Input: part model. Units: mm. Frame: model coordinates. A direction names the side the tool comes from. Coordinates: 2 decimals unless noted, no trailing zeros. Order: outer loops, then holes, each group sorted by start corner. A loop starts at its lowest first (then second) coordinate and runs counter-clockwise, first axis right, second up. Notation, with made-up numbers: (80.5, 32) - (139.5, 32) arc R36 ccw to (139.5, 67) - close; hole circle Ø10 at (61.25, 10). An arc over 180 degrees is marked (long way). Answer as CSV lines item,"result". Start each with the question number.
Item 1: Draft query along X for faces 6 (the cylindrical face through (-16.786, -0.592, 23.806)), 7 (the flat face through (-15, -1, 6.658)), 8 (the flat face through (-14.317, -1, 10)). Return one class per face: +X half, -X half, draft (parallel to the pull), parting line (faces both ways), or undercut.
Item 2: Section A-A (z = 11). Output: boundary loops of the cut face in (x, y).
Item 3: First-contact query: pin 1 (2 mm diameter, centred on y = -10.5, z = 27.5, fed in from +X); pin 2 (1 mm diameter, centred on x = -16.5, y = -1, fed in from +Z); pin 3 (1 mm diameter, centred on y = -0.5, z = 15, fed in from +X). Flat tips, straight axial feed; report the tip coordinate or a pass-through.
Item 4: Access query for faces 1 (the flat face through (-25, -1, 12.433)), 2 (the flat face through (-19, 0, 20)), 3 (the flat face through (-22.559, -1, 16)), 4 (the flat face through (-25, -1, 13.533)), 5 (the flat face through (-15.417, -1, 10)). Directions: +Z, -Z, +X, -X, +Y, -Y. A direction counts if a zero-diameter tool reaches every point of the face in a straight line with its end or side. Return the directions, or none.
Item 5: Section C-C (x = -23.25). Output: boundary loops of the cut face in (y, z).
Item 6: Material intervals for line 1 along X through (y, z) = (-1, 22.75); line 2 along X through (y, z) = (-1, 28.25); line 3 along Y through (x, z) = (-20.5, 22.5), sorted ascending.
Item 7: Section D-D (z = 22). Output: boundary loops of the cut face in (x, y).
Item 8: Section B-B (x = -18). Output: boundary loops of the cut face in (y, z), and give its area (3 significant figures).
from build123d import *

# Parameters (mm, degrees)
F1_DEPTH = 1.2
F2_R     = 0.267864
F3_DEPTH = 12.7


with BuildPart() as f1:
    # F0 (on Front) → F1 (new body)
    with BuildSketch(Plane.XZ):
        with BuildLine():
            Line((-22.558661, 13.532754), (-22.558661, 17.550706))
            ThreePointArc((-22.558661, 17.550706), (-20.646676, 18.025718), (-18.973681, 19.066109))
            ThreePointArc((-18.973681, 19.066109), (-17.31198, 18.043084), (-15.41748, 17.575431))
            Line((-15.41748, 17.575431), (-15.41748, 13.55748))
            Line((-15.41748, 13.55748), (-18.455535, 13.55748))
            Line((-18.455535, 13.55748), (-18.455535, 12.45748))
            Line((-18.455535, 12.45748), (-15.41748, 12.45748))
            Line((-15.41748, 12.45748), (-15.41748, 6.657985))
            Line((-15.41748, 6.657985), (-14.31748, 6.657985))
            Line((-14.31748, 6.657985), (-14.31748, 12.45748))
            Line((-14.31748, 12.45748), (-11.279425, 12.45748))
            Line((-11.279425, 12.45748), (-11.279425, 13.55748))
            Line((-11.279425, 13.55748), (-14.31748, 13.55748))
            Line((-14.31748, 13.55748), (-14.31748, 17.575431))
            ThreePointArc((-14.31748, 17.575431), (-9.043176, 26.336733), (-19.002461, 28.658661))
            ThreePointArc((-19.002461, 28.658661), (-28.940326, 26.294523), (-23.658661, 17.550706))
            Line((-23.658661, 17.550706), (-23.658661, 13.532754))
            Line((-23.658661, 13.532754), (-26.696716, 13.532754))
            Line((-26.696716, 13.532754), (-26.696716, 12.432754))
            Line((-26.696716, 12.432754), (-23.658661, 12.432754))
            Line((-23.658661, 12.432754), (-23.658661, 6.63326))
            Line((-23.658661, 6.63326), (-22.558661, 6.63326))
            Line((-22.558661, 6.63326), (-22.558661, 12.432754))
            Line((-22.558661, 12.432754), (-19.520607, 12.432754))
            Line((-19.520607, 12.432754), (-19.520607, 13.532754))
            Line((-19.520607, 13.532754), (-22.558661, 13.532754))
        make_face()
        with BuildLine():
            ThreePointArc((-19.634369, 19.720153), (-28.505536, 23.833831), (-19.659213, 28.000664))
            ThreePointArc((-19.659213, 28.000664), (-21.190733, 23.855777), (-19.634369, 19.720153))
        make_face(mode=Mode.SUBTRACT)
        with BuildLine():
            ThreePointArc((-18.977614, 20.377132), (-20.264355, 23.858556), (-18.998527, 27.347639))
            ThreePointArc((-18.998527, 27.347639), (-17.711786, 23.866214), (-18.977614, 20.377132))
        make_face(mode=Mode.SUBTRACT)
        with BuildLine():
            ThreePointArc((-18.341772, 28.004617), (-9.470605, 23.89094), (-18.316929, 19.724106))
            ThreePointArc((-18.316929, 19.724106), (-16.785408, 23.868994), (-18.341772, 28.004617))
        make_face(mode=Mode.SUBTRACT)
    extrude(amount=F1_DEPTH)

    # F2 (on face) → F3 (join)
    with BuildSketch(Plane.XZ.offset(1.2)):
        with Locations((-19.03018, 28.004617)):
            Circle(F2_R)
    extrude(amount=F3_DEPTH)


solid = f1.part
Determined:
1,face 6,"undercut"
1,face 7,"draft"
1,face 8,"+X half"
2,outline,"(-23.66, -1.2) - (-22.56, -1.2) - (-22.56, 0) - (-23.66, 0) - close; (-15.42, -1.2) - (-14.32, -1.2) - (-14.32, 0) - (-15.42, 0) - close"
3,pin 1,"stops at x = -18.76"
3,pin 2,"stops at z = 30.1"
3,pin 3,"stops at x = -14.32"
4,face 1,"-Z, -X, +Y, -Y"
4,face 2,"+Z, -Z, +X, -X, +Y"
4,face 3,"+Y, -Y"
4,face 4,"-X, +Y, -Y"
4,face 5,"-Z, +Y, -Y"
5,outline,"(-1.2, 6.63) - (0, 6.63) - (0, 18.45) - (-1.2, 18.45) - close; (-1.2, 29.25) - (0, 29.25) - (0, 30.17) - (-1.2, 30.17) - close"
6,line 1,"x = -29.34 to -28.39, -21.09 to -20.15, -17.83 to -16.88, -9.59 to -8.65"
6,line 2,"x = -27.65 to -26.23, -19.98 to -18.03, -11.71 to -10.3"
6,line 3,"y = -1.2 to 0"
7,outline,"(-29.16, -1.2) - (-28.18, -1.2) - (-28.18, 0) - (-29.16, 0) - close; (-20.91, -1.2) - (-19.93, -1.2) - (-19.93, 0) - (-20.91, 0) - close; (-18.04, -1.2) - (-17.06, -1.2) - (-17.06, 0) - (-18.04, 0) - close; (-9.81, -1.2) - (-8.83, -1.2) - (-8.83, 0) - (-9.81, 0) - close"
8,outline,"(-1.2, 12.46) - (0, 12.46) - (0, 13.56) - (-1.2, 13.56) - close; (-1.2, 18.38) - (0, 18.38) - (0, 19.48) - (-1.2, 19.48) - close; (-1.2, 20.12) - (0, 20.12) - (0, 22.11) - (-1.2, 22.11) - close; (-1.2, 25.59) - (0, 25.59) - (0, 27.58) - (-1.2, 27.58) - close; (-1.2, 28.27) - (0, 28.27) - (0, 29.37) - (-1.2, 29.37) - close"
8,area,"8.72 mm^2"
